from build123d import *

# Parameters (mm, degrees)
P_IDAT_VYSUNUT_M1_DEPTH  = 3
P_IDAT_VYSUNUT_M2_DEPTH  = 2
ZAOBLIT1_R               = 1
ZAOBLIT2_R               = 1
SKICA2_W                 = 4
SKICA2_H                 = 2
ODEBRAT_VYSUNUT_M1_DEPTH = 0.8


with BuildPart() as part:
    # Skica1 → P_idat vysunut_m1 (new body)
    with BuildSketch(Plane(origin=(0, 0, 0), x_dir=(1, 0, 0), z_dir=(0, 1, 0))):
        Polygon((118.524103266, 46.190077074), (105.53372221, 53.690077074), (103.593400635, 42.685966604), (92.248467845, 49.235966604), (102.473720104, 66.946623035), (91.301992395, 73.396623035), (89.463213481, 62.968389614), (78.635106664, 69.22), (39.317553332, 46.52), (0, 69.22), (0, 33.55662508), (-9.950504516, 37.17831254), (-9.950504516, 24.27831254), (10.5, 24.27831254), (10.5, 11.17831254), (0, 15), (0, 0), (15, 0), (55.910618513, 43.889876884), (111.018549767, 33.190077074), align=None)
    extrude(amount=P_IDAT_VYSUNUT_M1_DEPTH)

    # Skica1_3 → P_idat vysunut_m2 (add)
    with BuildSketch(Plane(origin=(0, 0, 0), x_dir=(1, 0, 0), z_dir=(0, 1, 0))):
        Polygon((91.856249834, 0), (111.018549767, 33.190077074), (55.910618513, 43.889876884), (15, 0), align=None)
    extrude(amount=P_IDAT_VYSUNUT_M2_DEPTH)

    # Zaoblit1
    zaoblit1_edges = [part.edges().sort_by_distance(p)[0] for p in [
        (102.473720104, 1.5, -66.946623035),
        (92.248467845, 1.5, -49.235966604),
        (103.593400635, 1.5, -42.685966604),
        (105.53372221, 1.5, -53.690077074),
        (0, 1.5, -15),
        (10.5, 1.5, -11.17831254),
        (10.5, 1.5, -24.27831254),
        (-9.950504516, 1.5, -24.27831254),
        (-9.950504516, 1.5, -37.17831254),
        (0, 1.5, -33.55662508),
        (89.463213481, 1.5, -62.968389614),
        (91.301992395, 1.5, -73.396623035),
    ]]
    fillet(zaoblit1_edges, radius=ZAOBLIT1_R)

    # Zaoblit2
    zaoblit2_edges = [part.edges().sort_by_distance(p)[0] for p in [
        (91.856249834, 1, 0),
    ]]
    fillet(zaoblit2_edges, radius=ZAOBLIT2_R)

    # Skica2 → Odebrat vysunut_m1 (cut)
    with BuildSketch(Plane(origin=(0, 3, 0), x_dir=(1, 0, 0), z_dir=(0, 1, 0))):
        with Locations((-7.950504516, 32.814238537)):
            Rectangle(SKICA2_W, SKICA2_H)
        with Locations((-7.950504516, 28.214238537)):
            Rectangle(SKICA2_W, SKICA2_H)
        Polygon((94.877656883, 47.718003606), (96.60970769, 46.718003606), (94.60970769, 43.253901991), (92.877656883, 44.253901991), align=None)
    extrude(amount=-ODEBRAT_VYSUNUT_M1_DEPTH, mode=Mode.SUBTRACT)


solid = part.part
Could you check a few things on this model? Use its own coordinates, in mm. A direction names the side the tool comes from. Round coordinates to 2 decimals unless told otherwise and drop trailing zeros. Order: outer loops, then holes, each group sorted by start corner. A loop starts at its lowest first (then second) coordinate and runs counter-clockwise, first axis right, second up.
Q1. Please list where these lines run through material, in increasing order: probe 1 along X at (y, z) = (0.55, -48); probe 2 along X at (y, z) = (2.2, -50.5); probe 3 along Y at (x, z) = (78, -13.5).
Geometry says:
probe 1: x = 0 to 36.75, 41.88 to 94.39, 104.53 to 115.39
probe 2: x = 0 to 32.42, 46.21 to 92.98, 104.97 to 111.06
probe 3: y = 0 to 2
Q2. Imagine slicing it at B-B, the plane z = -57.5. List the corners of the cut face in (x, y) for me.
Geometry says:
outline: (0, 0) - (20.3, 0) - (20.3, 3) - (0, 3) - close; (58.34, 0) - (97.02, 0) - (97.02, 3) - (58.34, 3) - close
Q3. Imagine slicing it at D-D, the plane z = -39.5. List the corners of the cut face in (x, y) for me, then the cut area to 3 significant figures.
Geometry says:
outline: (0, 0) - (114.66, 0) - (114.66, 3) - (78.52, 3) - (78.52, 2) - (51.82, 2) - (51.82, 3) - (0, 3) - close
area: 317 mm2
Q4. I'm going to push flat-ended pins straight in: P1, Ø0.9, axis at y = 2.5, z = -33, coming from the -X side; P2, Ø0.6, axis at x = -8.5, y = 3, coming from the +Z side; P3, Ø0.6, axis at x = -8, z = -28.5, coming from the +Y side; P4, Ø0.9, axis at y = 1.5, z = -18, coming from the -X side. Where does each tip first touch, or does it pass through?
Geometry says:
P1: stops at x = -9.95
P2: stops at z = -24.28
P3: stops at y = 2.2
P4: stops at x = 10.5
Q5. Thinking about a two-plate mould opening in X: for faces 1 (the face through (0, 1, -7)), 2 (the face through (53, 0, -29)), 3 (the face through (97.8, 1.48, -46.03)), which applies, released by +X, released by -X, zero draft, split by the parting line, or undercut?
Geometry says:
face 1: released by -X
face 2: zero draft
face 3: undercut
Q6. Imagine slicing it at C-C, the plane x = 71. List the corners of the cut face in (y, z) for me.
Geometry says:
outline: (0, -64.81) - (3, -64.81) - (3, -40.96) - (2, -40.96) - (2, 0) - (0, 0) - close
Q7. Which directions (+Z, -Z, +X, -X, +Y, -Y) give clear straight access to the entire face, cutting with the end or side of a thin tool? Please do faces 4 (the face through (90.392, 1.479, -68.236)), 5 (the face through (5.3, 1.48, -13.07)), 6 (the face through (83.079, 2.493, -38.615)), 7 (the face through (0, 1, -24.278)).
Geometry says:
face 4: -Z, +Y, -Y
face 5: +Y, -Y
face 6: +Z, +Y
face 7: -X, +Y, -Y
